Verification items for this drawing (mm, ordinates from the low corner). A direction names the side the tool comes from. Coordinates: 2 decimals unless noted, no trailing zeros. Loops run counter-clockwise (first coordinate to the right, second up) from the corner with the lowest first, then second, coordinate; pieces in that order, holes last. Notation, with made-up numbers: M 15.25,17.5 L 74.25,17.5 A17 cw 74.25,33.5 Z; hole C -33,48 d10. An arc over 180 degrees is marked long. Return JSON: item names as keys, results as strings.
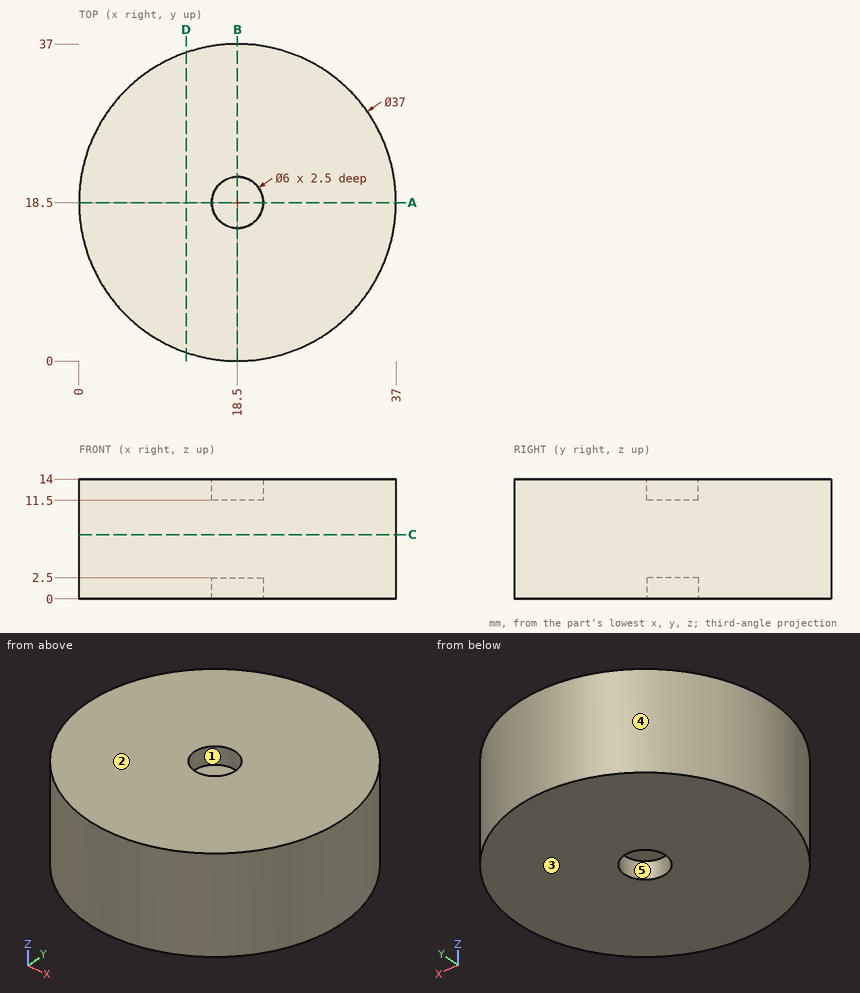
1) Section check D-D on x = 12.5. Record the cut outline in (y, z), then the cut area to 3 significant figures.
Answers:
{"outline": "M 1,0 L 36,0 L 36,14 L 1,14 Z", "area": "490 mm²"}
2) Scan lines: line 1 along Y through (x, z) = (18.5, 1.3); line 2 along X through (y, z) = (19, 9.25). Record each from-to range of solid material in increasing order. Write a range as [from, to].
Answers:
{"line 1": "[0, 15.5], [21.5, 37]", "line 2": "[0.01, 36.99]"}
3) Set-up check for the marked faces 1 and 2: record each of +Z, -Z, +X, -X, +Y, -Y from which the full face is reachable in a straight line by a thin tool's end or side.
Answers:
{"face 1": "+Z", "face 2": "+Z, +X, -X, +Y, -Y"}
4) Go/stop test with flat-tipped pins: pin 1 Ø3 at (x, y) = (17.5, 18) entering from +Z; pin 2 Ø3 at (x, y) = (12.5, 15) entering from -Z; pin 3 Ø6 at (y, z) = (32, 11.5) entering from +X; pin 4 Ø1 at (y, z) = (22.5, 10.5) entering from -X. Record where each tip stops, or that it passes through.
Answers:
{"pin 1": "z = 11.5", "pin 2": "z = 0", "pin 3": "x = 33.73", "pin 4": "x = 0.33"}
5) Section check A-A on y = 18.5. Record the cut outline in (x, z), then the cut area to 3 significant figures.
Answers:
{"outline": "M 0,0 L 15.5,0 L 15.5,2.5 L 21.5,2.5 L 21.5,0 L 37,0 L 37,14 L 21.5,14 L 21.5,11.5 L 15.5,11.5 L 15.5,14 L 0,14 Z", "area": "488 mm²"}
6) Section check C-C on z = 7.5. Record the cut outline in (x, y), then the cut area to 3 significant figures.
Answers:
{"outline": "C 18.5,18.5 d37", "area": "1,080 mm²"}
7) Draft check along X on the marked faces 3, 4 and 5. Enter one of: +X half, -X half, draft (parallel to the pull), parting line (faces both ways), or undercut.
Answers:
{"face 3": "draft", "face 4": "parting line", "face 5": "undercut"}
